Verification items for this drawing (mm, ordinates from the low corner). A direction names the side the tool comes from. Round coordinates to 2 decimals unless told otherwise and drop trailing zeros. Write each loop counter-clockwise with the first axis right and the second up, starting at its lowest first coordinate (ties: lowest second). Pieces come first, ordered by that corner, then holes. Notation, with made-up numbers: (40, 31) -> (51, 31) arc R21 ccw to (51, 70) -> close; hole circle Ø6 at (7.25, 16.25). An arc over 180 degrees is marked (long way). Put each result on its own line as item: value. Start each with the question number.
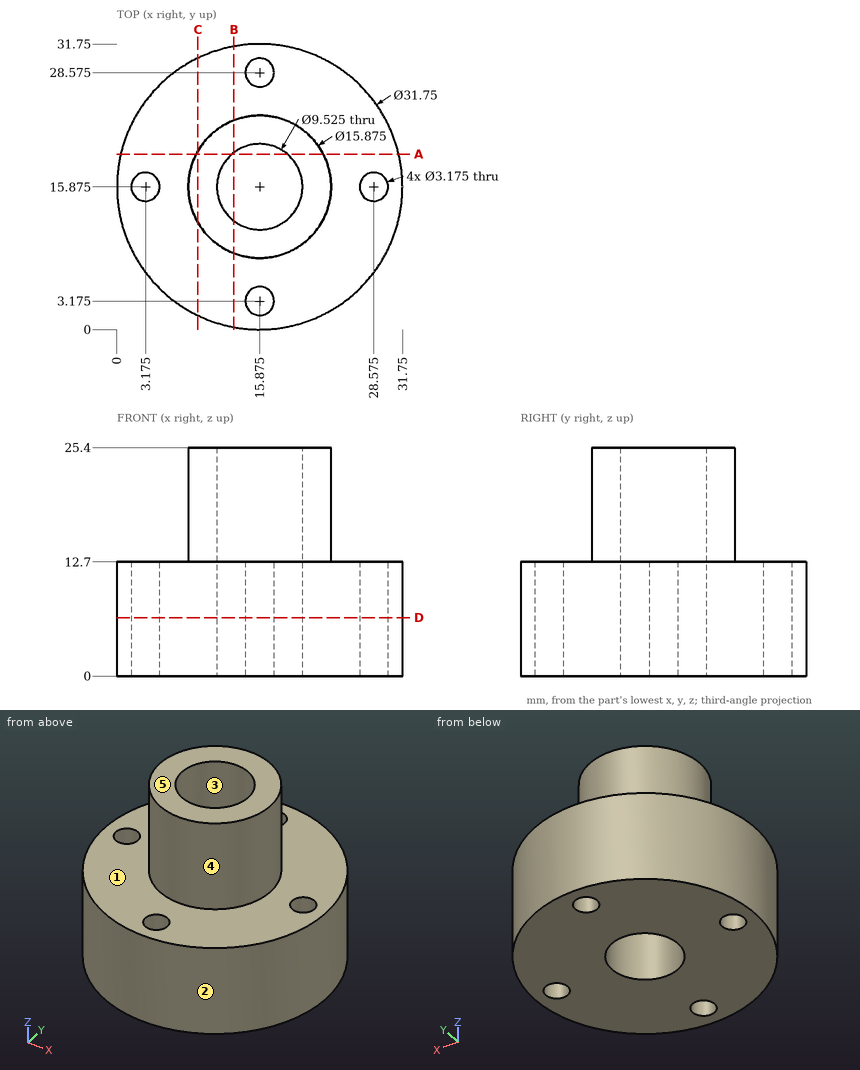
1. Material ranges on L1, parallel to Z at x = 7, y = 24; L2, parallel to Y at x = 18, z = 4; L3, parallel to X at y = 14.5, z = 15.5, recorded low to high. Write a range as [from, to].
2. Draft check along X on the marked faces 1, 2 and 3. Enter one of: released by +X, released by -X, zero draft, split by the parting line, or undercut.
3. Section check A-A, the plane y = 19.5. Enter the section's corners in (x, z).
4. Section check D-D, the plane z = 6.5. Give the number of separate pieces and of enclosed holes in the cut face, then the cut area to 3 significant figures.
5. Section check C-C, the plane x = 9. Enter the section's corners in (y, z), then the cut area to 3 significant figures.
6. Gauge pin test, flat ends, axial feed: P1, Ø5, axis at x = 28.575, y = 15.875, coming from the +Z side; P2, Ø5, axis at x = 13.5, z = 11.5, coming from the +Y side; P3, Ø3, axis at x = 15.875, y = 3.175, coming from the -Z side; P4, Ø1.5, axis at y = 12.5, z = 20, coming from the +X side. Record the tip position at first contact, or that the pin passes through.
7. Access from +Z, -Z, +X, -X, +Y, -Y to the whole of each face (thin tool, end or side, straight path). Record for the marked faces 4 and 5.
8. Section check B-B, the plane x = 13. Enter the section's corners in (y, z), then the cut area to 3 significant figures.
Reply:
1. L1: z = [0, 12.7]
1. L2: y = [0.14, 11.61], [20.14, 31.61]
1. L3: x = [8.06, 11.32], [20.43, 23.69]
2. face 1: zero draft
2. face 2: split by the parting line
2. face 3: undercut
3. outline: (0.42, 0) -> (12.79, 0) -> (12.79, 25.4) -> (8.81, 25.4) -> (8.81, 12.7) -> (0.42, 12.7) -> close; (18.96, 0) -> (31.33, 0) -> (31.33, 12.7) -> (22.94, 12.7) -> (22.94, 25.4) -> (18.96, 25.4) -> close
4. separate pieces: 1
4. enclosed holes: 5
4. area: 689 mm2
5. outline: (1.57, 0) -> (30.18, 0) -> (30.18, 12.7) -> (19.84, 12.7) -> (19.84, 25.4) -> (11.91, 25.4) -> (11.91, 12.7) -> (1.57, 12.7) -> close
5. area: 464 mm2
6. P1: stops at z = 12.7
6. P2: stops at y = 31.75
6. P3: passes through
6. P4: stops at x = 23.37
7. face 4: +Z
7. face 5: +Z, +X, -X, +Y, -Y
8. outline: (0.26, 0) -> (12.08, 0) -> (12.08, 25.4) -> (8.48, 25.4) -> (8.48, 12.7) -> (0.26, 12.7) -> close; (19.67, 0) -> (31.49, 0) -> (31.49, 12.7) -> (23.27, 12.7) -> (23.27, 25.4) -> (19.67, 25.4) -> close
8. area: 392 mm2
